Read the model definition and answer for the solid it produces. Units are mm, in the model's axes. Face numbers are marked on the shaded views. A direction names the side the tool comes from. Round coordinates to 2 decimals unless told otherwise and drop trailing zeros. Order: outer loops, then holes, each group sorted by start corner. A loop starts at its lowest first (then second) coordinate and runs counter-clockwise, first axis right, second up. Notation, with made-up numbers: (64.25, -17) -> (91.25, -17) arc R18 ccw to (91.25, 16) -> close; hole circle Ø5 at (2.5, 49.5). An arc over 180 degrees is marked (long way). Answer as a JSON object with one key per item and string values. Group by question number.
Item 1: The mould has two halves that part along X. Classify the marked faces 4, 5 and 6: pulls with the +X half, pulls with the -X half, needs draft (parallel to the pull), parting line crosses it, or undercut.
Item 2: Given P1, Ø2, axis at y = 4, z = -0.5, coming from the -X side; P2, Ø1, axis at x = 0.5, z = -0.5, coming from the -Y side; P3, Ø1.5, axis at x = 0.5, y = 2, coming from the +Z side, each flat-ended and moving along its own axis, determine where each tip first touches the part or whether it passes through.
Item 3: For the marked faces 1, 2 and 3, determine the directions among +Z, -Z, +X, -X, +Y, -Y from which every point of the face is accessible in a straight line to the end or side of a thin tool.
Item 4: Section B-B, the plane x = 0.2 is taken. Write down the section's boundary in (y, z).
Item 5: Section C-C, the plane y = 3 is taken. Write down the section's boundary in (x, z).
Item 6: Section D-D, the plane y = -0.5 is taken. Write down the section's boundary in (x, z).
Item 7: Consider probe 1 along Y at (x, z) = (-0.5, 1.05); probe 2 along Y at (x, z) = (-0.65, 2); probe 3 along Z at (x, y) = (-0.95, -1.5). Determine where each line is inside the solid, lowest interval first. Write a range as from..to.
Item 8: Section A-A, the plane z = 0 is taken. Write down the section's boundary in (x, y), plus the area to 3 significant figures.
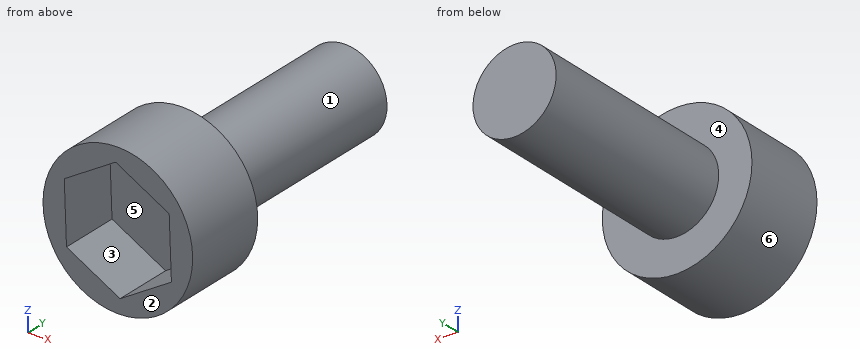
from build123d import *

# Parameters (mm, degrees)
SKETCH1_R           = 1.27
BOSS_EXTRUDE1_DEPTH = 6.35
SKETCH2_R           = 2.286
BOSS_EXTRUDE2_DEPTH = 2.54
CUT_EXTRUDE1_DEPTH  = 1.778


with BuildPart() as part:
    # Sketch1 → Boss-Extrude1 (new body)
    with BuildSketch(Plane(origin=(0, 0, 0), x_dir=(1, 0, 0), z_dir=(0, 1, 0))):
        with Locations(Location((0, 0, 0), (0, 0, 270))):
            Circle(SKETCH1_R)
    extrude(amount=BOSS_EXTRUDE1_DEPTH)

    # Sketch2 → Boss-Extrude2 (add)
    with BuildSketch(Plane.XZ):
        with Locations(Location((0, 0, 0), (0, 0, 270))):
            Circle(SKETCH2_R)
    extrude(amount=BOSS_EXTRUDE2_DEPTH)

    # Sketch3 → Cut-Extrude1 (cut)
    with BuildSketch(Plane(origin=(0, -2.54, 0), x_dir=(-1, 0, 0), z_dir=(0, -1, 0))):
        Polygon((-0.068044734, 1.850241436), (-1.636378453, 0.86619225), (-1.56833372, -0.984049186), (0.068044734, -1.850241436), (1.636378453, -0.86619225), (1.56833372, 0.984049186), align=None)
    extrude(amount=-CUT_EXTRUDE1_DEPTH, mode=Mode.SUBTRACT)


solid = part.part
Values found:
{
 "1": {"face 4": "needs draft", "face 5": "undercut", "face 6": "parting line crosses it"},
 "2": {"P1": "x = -1.27", "P2": "y = -0.76", "P3": "z = 1.27"},
 "3": {"face 1": "+Y", "face 2": "+Z, -Z, +X, -X, -Y", "face 3": "-Y"},
 "4": {"outline": "(-2.54, -2.28) -> (0, -2.28) -> (0, -1.25) -> (6.35, -1.25) -> (6.35, 1.25) -> (0, 1.25) -> (0, 2.28) -> (-2.54, 2.28) -> (-2.54, 1.71) -> (-0.76, 1.71) -> (-0.76, -1.77) -> (-2.54, -1.77) -> close"},
 "5": {"outline": "circle Ø2.54 at (0, 0)"},
 "6": {"outline": "circle Ø4.57 at (0, 0)"},
 "7": {"probe 1": "-0.76..6.35", "probe 2": "-2.54..0", "probe 3": "-2.08..-1.31, 1.3..2.08"},
 "8": {"outline": "(-2.29, -2.54) -> (-1.6, -2.54) -> (-1.6, -0.76) -> (1.6, -0.76) -> (1.6, -2.54) -> (2.29, -2.54) -> (2.29, 0) -> (1.27, 0) -> (1.27, 6.35) -> (-1.27, 6.35) -> (-1.27, 0) -> (-2.29, 0) -> close", "area": "22.0 mm2"}
}
